CAD build for the part. Positions are in the model's coordinates, mm. A direction names the side the tool comes from. Round coordinates to 2 decimals unless told otherwise and drop trailing zeros. Write each loop counter-clockwise with the first axis right and the second up, starting at its lowest first coordinate (ties: lowest second). Pieces come first, ordered by that corner, then holes. Notation, with made-up numbers: M 55,45.25 L 83,45.25 A9 cw 83,58.25 Z; hole C 10,45 d1. An arc over 180 degrees is marked long. Write each question's results on one line, items separated by ' | '. Start each with the question number.
```python
from build123d import *
from OCP.BRepFilletAPI import BRepFilletAPI_MakeFillet

# Parameters (mm, degrees)
BOSS_EXTRUDE1_DEPTH = 3
FILLET1_R1          = 10
FILLET1_R2          = 5
SKETCH2_R           = 2.5
CUT_EXTRUDE1_DEPTH  = 56.768397029


with BuildPart() as part:
    # Sketch1 → Boss-Extrude1 (new body)
    with BuildSketch(Plane(origin=(0, 0, 0), x_dir=(1, 0, 0), z_dir=(0, 1, 0))):
        Polygon((-20, 0), (20, 0), (20, 30), (0, 60), (-20, 30), align=None)
    extrude(amount=BOSS_EXTRUDE1_DEPTH)

    # Fillet1: one fillet with a radius per group of edges: ONE call of the kernel's fillet builder (fillet() takes one radius for all edges)
    fillet1_edges_1 = [part.edges().sort_by_distance(p)[0] for p in [
        (20, 1.5, -30),
        (-20, 1.5, -30),
        (0, 1.5, -60),
    ]]
    fillet1_edges_2 = [part.edges().sort_by_distance(p)[0] for p in [
        (20, 1.5, 0),
        (-20, 1.5, 0),
    ]]
    fillet1 = BRepFilletAPI_MakeFillet(part.part.solid().wrapped)
    for e in fillet1_edges_1:
        fillet1.Add(FILLET1_R1, e.wrapped)
    for e in fillet1_edges_2:
        fillet1.Add(FILLET1_R2, e.wrapped)
    add(Compound.cast(fillet1.Shape()), mode=Mode.REPLACE)

    # Sketch2 → Cut-Extrude1 (cut, through all)
    with BuildSketch(Plane(origin=(0, 3, 0), x_dir=(1, 0, 0), z_dir=(0, 1, 0))):
        with Locations(Location((0, 35, 0), (0, 0, 270))):
            Circle(SKETCH2_R)
        with BuildLine():
            Line((-12.5, 12), (12.5, 12))
            ThreePointArc((12.5, 12), (14.5, 10), (12.5, 8))
            Line((12.5, 8), (-12.5, 8))
            ThreePointArc((-12.5, 8), (-14.5, 10), (-12.5, 12))
        make_face()
    extrude(amount=-CUT_EXTRUDE1_DEPTH, mode=Mode.SUBTRACT)


solid = part.part
```
1) Saw through at A-A, the plane z = -10. Write the cut outline in (x, y).
2) Saw through at D-D, the plane z = -35. Write the cut outline in (x, y).
3) Saw through at C-C, the plane x = 0. Write the cut outline in (y, z), plus the area to 3 significant figures.
4) Wall check: line 1 along Z through (x, y) = (-8, 2.6); line 2 along X through (y, z) = (1.5, -35); line 3 along X through (y, z) = (0.5, -11). Give the ranges that are in metal, low to high. Write a range as from..to.
5) Drop flat-ended pins along their axis: pin 1 Ø1.5 at (x, z) = (11, -25) entering from -Y; pin 2 Ø3 at (x, z) = (0, -35) entering from +Y. Give the stop position or say it passes through.
6) Saw through at B-B, the plane y = 0.7. Write the cut outline in (x, z), plus the area to 3 significant figures.
7) 3-axis set-ups, long thin cutter, end or side, ignore diameter. For faces 1 (the face through (20, 1, -16)), 2 (the face through (0, 2, -8)): which of +Z, -Z, +X, -X, +Y, -Y reach the whole face in a straight line?
8) Pull direction Z, two halves, no side cores. Call faces 3 (the face through (18, 2, -1)), 4 (the face through (13.4, 1.5, -39.9)), 5 (the face through (-14.5, 1.5, -10)): pulls with the +Z half, pulls with the -Z half, needs draft (parallel to the pull), parting line crosses it, or undercut.
Filled sheet:
1) outline: M -20,0 L -14.5,0 L -14.5,3 L -20,3 Z; M 14.5,0 L 20,0 L 20,3 L 14.5,3 Z
2) outline: M -16.67,0 L -2.5,0 L -2.5,3 L -16.67,3 Z; M 2.5,0 L 16.67,0 L 16.67,3 L 2.5,3 Z
3) outline: M 0,-51.97 L 3,-51.97 L 3,-37.5 L 0,-37.5 Z; M 0,-32.5 L 3,-32.5 L 3,-12 L 0,-12 Z; M 0,-8 L 3,-8 L 3,0 L 0,0 Z | area: 129 mm^2
4) line 1: z = -47.97..-12, -8..0 | line 2: x = -16.67..-2.5, 2.5..16.67 | line 3: x = -20..-14.23, 14.23..20
5) pin 1: stops at y = 0 | pin 2: passes through
6) outline: M -20,-26.97 A10 ccw -18.32,-32.52 L -8.32,-47.52 A10 ccw 8.32,-47.52 L 18.32,-32.52 A10 ccw 20,-26.97 L 20,-5 A5 ccw 15,0 L -15,0 A5 ccw -20,-5 Z; hole M -12.5,-12 L 12.5,-12 A2 ccw 12.5,-8 L -12.5,-8 A2 ccw Z; hole C 0,-35 d5 | area: 1,600 mm^2
7) face 1: +Z, -Z, +X, +Y, -Y | face 2: +Y, -Y
8) face 3: pulls with the +Z half | face 4: pulls with the -Z half | face 5: undercut
